Design review of the part built by this model. Coordinates are the model's own, in mm. A direction names the side the tool comes from. Give positions to 0.01 mm unless a question says otherwise; leave off trailing zeros. Order: outer loops, then holes, each group sorted by start corner. A loop starts at its lowest first (then second) coordinate and runs counter-clockwise, first axis right, second up. Notation, with made-up numbers: M 4,-24 L 11,-24 A14 cw 11,-7 Z; hole C 62,-21 d5. An arc over 180 degrees is marked long. Put each result on its own line as item: value. Start each with the question number.
from build123d import *

# Parameters (mm, degrees)
ESQUISSE1_W             = 39
ESQUISSE1_H             = 64
ESQUISSE1_R             = 2.5
BOSS_EXTRU_1_DEPTH      = 5
ESQUISSE2_W             = 5
ESQUISSE2_H             = 64
BOSS_EXTRU_2_DEPTH      = 130
ESQUISSE3_R             = 19
ENL_V_MAT_EXTRU_1_DEPTH = 148.163174742
ESQUISSE4_W             = 5
ESQUISSE4_H             = 8
BOSS_EXTRU_3_DEPTH      = 52


with BuildPart() as part:
    # Esquisse1 → Boss.-Extru.1 (new body)
    with BuildSketch(Plane.XY):
        with Locations((-19.5, 32)):
            Rectangle(ESQUISSE1_W, ESQUISSE1_H)
        with Locations((-5.5, 51)):
            Circle(ESQUISSE1_R, mode=Mode.SUBTRACT)
        with Locations((-5.5, 27)):
            Circle(ESQUISSE1_R, mode=Mode.SUBTRACT)
    extrude(amount=BOSS_EXTRU_1_DEPTH)

    # Esquisse2 → Boss.-Extru.2 (add)
    with BuildSketch(Plane.XY.offset(5)):
        with Locations((-41.5, 32)):
            Rectangle(ESQUISSE2_W, ESQUISSE2_H)
    extrude(amount=-BOSS_EXTRU_2_DEPTH)

    # Esquisse3 → Enlèv. mat.-Extru.1 (cut, through all)
    with BuildSketch(Plane.ZY.offset(44)):
        with Locations(Location((-96.8, 33.8, 0), (0, 0, 270))):
            Circle(ESQUISSE3_R)
    extrude(amount=-ENL_V_MAT_EXTRU_1_DEPTH, mode=Mode.SUBTRACT)

    # Esquisse4 → Boss.-Extru.3 (add)
    with BuildSketch(Plane.ZY.offset(44)):
        with Locations((-74.5, 34)):
            Rectangle(ESQUISSE4_W, ESQUISSE4_H)
        with Locations((-119.5, 34)):
            Rectangle(ESQUISSE4_W, ESQUISSE4_H)
    extrude(amount=BOSS_EXTRU_3_DEPTH)


solid = part.part
1. The part is to be moulded in two halves that separate along Z. For faces 1 (the flat face through (-42, 32, -125)), 2 (the flat face through (-96, 34, -75)), 3 (the flat face through (-70, 34, -77)), 4 (the flat face through (-70, 34, -117)), say which applies: +Z half, -Z half, draft (parallel to the pull), parting line (faces both ways), or undercut.
2. Consider section D-D on x = -69.5. Give the boundary of the cut face in (y, z).
3. Insertion check: pin 1 (9 mm diameter, centred on x = -67.5, y = 35, fed in from +Z); pin 2 (1 mm diameter, centred on x = -36.5, y = 10, fed in from -Z); pin 3 (9 mm diameter, centred on x = -69.5, y = 35.5, fed in from -Z). Each pin has a flat end and moves straight along its axis. Give the tip position at first contact, or say it passes through.
4. Consider section A-A on z = -96.8. Give the boundary of the cut face in (x, y).
5. To check wall thickness, follow probe 1 along Y at (x, z) = (-5.5, 1.1); probe 2 along Z at (x, y) = (-71, 37.5); probe 3 along Z at (x, y) = (-42.05, 33.8). State the ranges of each line that lie inside material, in increasing order.
6. Consider section C-C on y = 33.8. Give the boundary of the cut face in (x, z).
7. Consider section B-B on x = -5.5. Give the boundary of the cut face in (y, z), then the cut area to 3 significant figures.
8. Machinability: for faces 5 (the flat face through (-70, 30, -75)), 6 (the flat face through (-70, 38, -75)), 7 (the flat face through (-70, 34, -122)), 8 (the flat face through (-39, 32, -62)), 9 (the flat face through (-96, 34, -120)), which of the approach directions +Z, -Z, +X, -X, +Y, -Y give a long, thin tool a straight path to every point of the face, cutting with its end or side? Answer none if there is none.
Returned:
1. face 1: -Z half
1. face 2: draft
1. face 3: undercut
1. face 4: undercut
2. outline: M 30,-122 L 38,-122 L 38,-117 L 30,-117 Z; M 30,-77 L 38,-77 L 38,-72 L 30,-72 Z
3. pin 1: stops at z = -72
3. pin 2: stops at z = 0
3. pin 3: stops at z = -122
4. outline: M -44,0 L -39,0 L -39,14.8 L -44,14.8 Z; M -44,52.8 L -39,52.8 L -39,64 L -44,64 Z
5. probe 1: y = 0 to 24.5, 29.5 to 48.5, 53.5 to 64
5. probe 2: z = -122 to -117, -77 to -72
5. probe 3: z = -125 to -115.8, -77.8 to 5
6. outline: M -96,-122 L -44,-122 L -44,-125 L -39,-125 L -39,-115.8 L -44,-115.8 L -44,-117 L -96,-117 Z; M -96,-77 L -44,-77 L -44,-77.8 L -39,-77.8 L -39,0 L 0,0 L 0,5 L -44,5 L -44,-72 L -96,-72 Z
7. outline: M 0,0 L 24.5,0 L 24.5,5 L 0,5 Z; M 29.5,0 L 48.5,0 L 48.5,5 L 29.5,5 Z; M 53.5,0 L 64,0 L 64,5 L 53.5,5 Z
7. area: 270 mm2
8. face 5: +Z, -Z, -X, -Y
8. face 6: +Z, -Z, -X, +Y
8. face 7: -Z, -X, +Y, -Y
8. face 8: -Z, +X, +Y, -Y
8. face 9: +Z, -Z, -X, +Y, -Y
